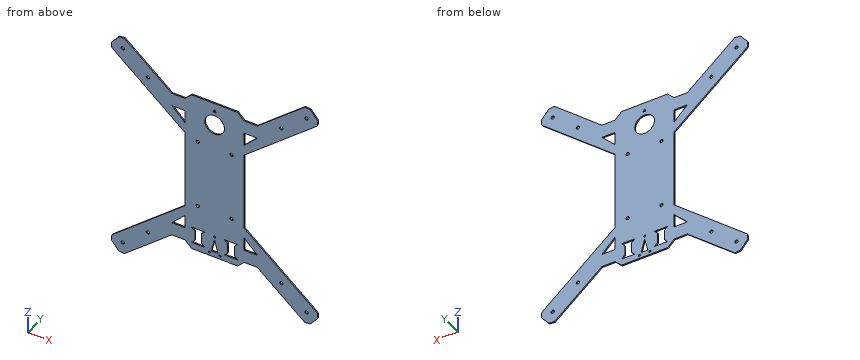
from build123d import *

# Parameters (mm, degrees)
Y_KSEKLIK_EKSTR_ZYON2_DEPTH = 2
KES_EKSTR_ZYON2_DEPTH       = 2
KES_EKSTR_ZYON3_DEPTH       = 20
PAH1_SIZE                   = 6
IZIM6_R                     = 2.5
KES_EKSTR_ZYON4_DEPTH       = 20
IZIM7_R                     = 1.55
KES_EKSTR_ZYON5_DEPTH       = 10
IZIM8_R                     = 15
KES_EKSTR_ZYON6_DEPTH       = 2
KES_EKSTR_ZYON7_DEPTH       = 10
KES_EKSTR_ZYON8_DEPTH       = 10
IZIM11_R                    = 2.5
KES_EKSTR_ZYON9_DEPTH       = 10


with BuildPart() as part:
    # Çizim2 → Yükseklik-Ekstrüzyon2 (new body)
    with BuildSketch(Plane(origin=(0, 0, 0), x_dir=(1, 0, 0), z_dir=(0, 1, 0))):
        Polygon((-160.888072602, 157.241638979), (-45, 60), (-45, -60), (-160.888072602, -157.241638979), (-141.604444312, -180.222972272), (-65, -115.944211304), (-45, -115.944211304), (-35, -125.944211304), (35, -125.944211304), (45, -115.944211304), (65, -115.944211304), (141.604444312, -180.222972272), (160.888072602, -157.241638979), (45, -60), (45, 60), (160.888072602, 157.241638979), (141.604444312, 180.222972272), (65, 115.944211304), (45, 115.944211304), (35, 125.944211304), (-35, 125.944211304), (-45, 115.944211304), (-65, 115.944211304), (-141.604444312, 180.222972272), align=None)
    extrude(amount=Y_KSEKLIK_EKSTR_ZYON2_DEPTH)

    # Çizim4 → Kes-Ekstrüzyon2 (cut)
    with BuildSketch(Plane(origin=(0, 2, 0), x_dir=(1, 0, 0), z_dir=(0, 1, 0))):
        Polygon((-2.5, -111.614084285), (0, -115.944211304), (2.5, -111.614084285), align=None)
    extrude(amount=-KES_EKSTR_ZYON2_DEPTH, mode=Mode.SUBTRACT)

    # Çizim5 → Kes-Ekstrüzyon3 (cut)
    with BuildSketch(Plane(origin=(0, 2, 0), x_dir=(1, 0, 0), z_dir=(0, 1, 0))):
        Polygon((-65, 95.944211304), (-45, 95.944211304), (-45, 75.944211304), align=None)
        Polygon((45, 75.944211304), (65, 95.944211304), (45, 95.944211304), align=None)
        Polygon((65, -95.944211304), (45, -95.944211304), (45, -75.944211304), align=None)
        Polygon((-45, -75.944211304), (-65, -95.944211304), (-45, -95.944211304), align=None)
    extrude(amount=-KES_EKSTR_ZYON3_DEPTH, mode=Mode.SUBTRACT)

    # Pah1
    pah1_edges = [part.edges().sort_by_distance(p)[0] for p in [
        (-160.888072602, 1, -157.241638979),
        (-141.604444312, 1, -180.222972272),
        (141.604444312, 1, -180.222972272),
        (160.888072602, 1, -157.241638979),
        (160.888072602, 1, 157.241638979),
        (141.604444312, 1, 180.222972272),
        (-141.604444312, 1, 180.222972272),
        (-160.888072602, 1, 157.241638979),
    ]]
    chamfer(pah1_edges, length=PAH1_SIZE)

    # Çizim6 → Kes-Ekstrüzyon4 (cut)
    with BuildSketch(Plane(origin=(0, 2, 0), x_dir=(1, 0, 0), z_dir=(0, 1, 0))):
        with Locations(Location((-139.75559181, 159.09049148, 0), (0, 0, 270))):
            Circle(IZIM6_R)
        with Locations(Location((-101.453369654, 126.951110996, 0), (0, 0, 270))):
            Circle(IZIM6_R)
        with Locations(Location((101.453369654, 126.951110996, 0), (0, 0, 270))):
            Circle(IZIM6_R)
        with Locations(Location((139.75559181, 159.09049148, 0), (0, 0, 270))):
            Circle(IZIM6_R)
        with Locations(Location((101.453369654, -126.951110996, 0), (0, 0, 270))):
            Circle(IZIM6_R)
        with Locations(Location((139.75559181, -159.09049148, 0), (0, 0, 270))):
            Circle(IZIM6_R)
        with Locations(Location((-101.453369654, -126.951110996, 0), (0, 0, 270))):
            Circle(IZIM6_R)
        with Locations(Location((-139.75559181, -159.09049148, 0), (0, 0, 270))):
            Circle(IZIM6_R)
    extrude(amount=-KES_EKSTR_ZYON4_DEPTH, mode=Mode.SUBTRACT)

    # Çizim7 → Kes-Ekstrüzyon5 (cut)
    with BuildSketch(Plane(origin=(0, 2, 0), x_dir=(1, 0, 0), z_dir=(0, 1, 0))):
        with Locations(Location((-8, 120.944211304, 0), (0, 0, 270))):
            Circle(IZIM7_R)
        with Locations(Location((8, 120.944211304, 0), (0, 0, 270))):
            Circle(IZIM7_R)
        with Locations(Location((0, 92.780546714, 0), (0, 0, 270))):
            Circle(IZIM7_R)
    extrude(amount=-KES_EKSTR_ZYON5_DEPTH, mode=Mode.SUBTRACT)

    # Çizim8 → Kes-Ekstrüzyon6 (cut)
    with BuildSketch(Plane(origin=(0, 2, 0), x_dir=(1, 0, 0), z_dir=(0, 1, 0))):
        with Locations(Location((0, -90.944211304, 0), (0, 0, 270))):
            Circle(IZIM8_R)
    extrude(amount=-KES_EKSTR_ZYON6_DEPTH, mode=Mode.SUBTRACT)

    # Çizim9 → Kes-Ekstrüzyon7 (cut)
    with BuildSketch(Plane(origin=(0, 2, 0), x_dir=(1, 0, 0), z_dir=(0, 1, 0))):
        Polygon((-35, 115.944211304), (-15, 115.944211304), (-20, 110.944211304), (-20, 95.944211304), (-15, 90.944211304), (-35, 90.944211304), (-30, 95.944211304), (-30, 110.944211304), align=None)
        Polygon((30, 110.944211304), (35, 115.944211304), (15, 115.944211304), (20, 110.944211304), (20, 95.944211304), (15, 90.944211304), (35, 90.944211304), (30, 95.944211304), align=None)
    extrude(amount=-KES_EKSTR_ZYON7_DEPTH, mode=Mode.SUBTRACT)

    # Çizim10 → Kes-Ekstrüzyon8 (cut)
    with BuildSketch(Plane(origin=(0, 2, 0), x_dir=(1, 0, 0), z_dir=(0, 1, 0))):
        Polygon((-5, 117.413602047), (0, 97.413602047), (5, 117.413602047), align=None)
    extrude(amount=-KES_EKSTR_ZYON8_DEPTH, mode=Mode.SUBTRACT)

    # Çizim11 → Kes-Ekstrüzyon9 (cut)
    with BuildSketch(Plane(origin=(0, 2, 0), x_dir=(1, 0, 0), z_dir=(0, 1, 0))):
        with Locations(Location((25.75, -52.5, 0), (0, 0, 270))):
            Circle(IZIM11_R)
        with Locations(Location((-25.75, -52.5, 0), (0, 0, 270))):
            Circle(IZIM11_R)
        with Locations(Location((-25.75, 52.5, 0), (0, 0, 270))):
            Circle(IZIM11_R)
        with Locations(Location((25.75, 52.5, 0), (0, 0, 270))):
            Circle(IZIM11_R)
    extrude(amount=-KES_EKSTR_ZYON9_DEPTH, mode=Mode.SUBTRACT)


solid = part.part
Verification items for the finished model (mm, model axes). Round coordinates to 2 decimals unless told otherwise and drop trailing zeros. Loops run counter-clockwise (first coordinate to the right, second up) from the corner with the lowest first, then second, coordinate; pieces in that order, holes last. Notation, with made-up numbers: (57.25, -31) - (66.25, -31) arc R13 cw to (66.25, -23) - close; hole circle Ø4 at (27, -9). An arc over 180 degrees is marked (long way). Write item = value, one per line.
Q1. Material ranges on L1, parallel to Z at x = -138, y = 0.3; L2, parallel to Z at x = 54.5, y = 1.4; L3, parallel to X at y = 1.1, z = -89.5, recorded low to high.
Here are the results:
L1 = -176.28 to -160.87, -157.31 to -138.04, 138.04 to 157.31, 160.87 to 176.28
L2 = -115.94 to -95.94, -85.44 to -67.97, 67.97 to 85.44, 95.94 to 115.94
L3 = -80.16 to -58.56, -45 to 45, 58.56 to 80.16
Q2. Sectioned sample at C-C on y = 1.5. State how many separate pieces and enclosed holes the cut face has, plus the area to 3 significant figures.
Here are the results:
separate_pieces = 1
enclosed_holes = 24
area = 37,200 mm^2
Q3. Sectioned sample at B-B on x = -76. Record the boundary of the cut face in (y, z), plus the area to 3 significant figures.
Here are the results:
outline = (0, -125.17) - (2, -125.17) - (2, -86.01) - (0, -86.01) - close; (0, 86.01) - (2, 86.01) - (2, 125.17) - (0, 125.17) - close
area = 157 mm^2
Q4. Sectioned sample at D-D on z = -35. Record the boundary of the cut face in (x, y).
Here are the results:
outline = (-45, 0) - (45, 0) - (45, 2) - (-45, 2) - close
Q5. Sectioned sample at A-A on z = -86.5. Record the boundary of the cut face in (x, y), plus the area to 3 significant figures.
Here are the results:
outline = (-76.58, 0) - (-55.56, 0) - (-55.56, 2) - (-76.58, 2) - close; (-45, 0) - (45, 0) - (45, 2) - (-45, 2) - close; (55.56, 0) - (76.58, 0) - (76.58, 2) - (55.56, 2) - close
area = 264 mm^2
Q6. Depth check by flat-ended pin: pin 1 (0.6 mm diameter, centred on x = 1.5, y = 1.5, fed in from +Z); pin 2 (0.6 mm diameter, centred on x = -51, y = 1.5, fed in from -Z); pin 3 (3 mm diameter, centred on x = -139.76, z = 159.09, fed in from +Y); pin 4 (1 mm diameter, centred on y = 1, z = -82, fed in from +X). Enter the tip coordinate at first touch or a pass-through.
Here are the results:
pin_1 = 125.94
pin_2 = -115.94
pin_3 = through
pin_4 = 71.81
